Work out the finished part from the listing and answer in its coordinate system (mm). Face numbers are marked on the shaded views. A direction names the side the tool comes from. Give positions to 0.01 mm unless a question says otherwise; leave off trailing zeros. Order: outer loops, then holes, each group sorted by start corner. A loop starts at its lowest first (then second) coordinate and runs counter-clockwise, first axis right, second up. Notation, with made-up numbers: (38.25, -17) -> (79.25, -17) arc R29 ccw to (79.25, 12) -> close; hole circle Ø1 at (56.25, 59.5). An arc over 180 degrees is marked (long way). Answer as CSV lines item,"result". Start each with the question number.
1. For the marked faces 5 and 6, determine the directions among +Z, -Z, +X, -X, +Y, -Y from which every point of the face is accessible in a straight line to the end or side of a thin tool.
2. A cutting plane is placed at C-C (y = 35.5). Give the vertices of the cut face in (x, z) (3 decimals).
3. A cutting plane is placed at D-D (y = -38). Give the vertices of the cut face in (x, z) (3 decimals), then the cut area to 3 significant figures.
4. Find the intervals of material crossed by L1, parallel to X at y = -3, z = -2; L2, parallel to X at y = -0.5, z = -1.5; L3, parallel to Y at x = 4, z = -0.75, in increasing order.
5. For a pull along Y with two mould halves and no side action, classify the marked faces 1, 2, 3 and 4 as released by +Y, released by -Y, zero draft, split by the parting line, or undercut.
6. A cutting plane is placed at A-A (x = 0). Give the vertices of the cut face in (y, z) (3 decimals).
7. Flat-ended cylindrical pins translate along their axes: pin 1 (2 mm diameter, centred on x = -25, z = 1, fed in from +Y); pin 2 (3 mm diameter, centred on x = -1.5, z = 0, fed in from -Y); pin 3 (2 mm diameter, centred on x = 1.5, z = 1, fed in from +Y). Find the tip coordinate at first contact, or state that the pin passes through.
8. A cutting plane is placed at B-B (z = 2). Give the vertices of the cut face in (x, y), then the cut area to 3 significant figures.
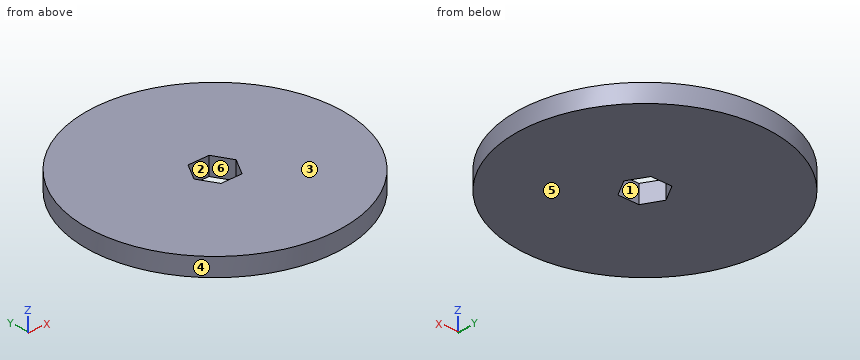
from build123d import *

# Parameters (mm, degrees)
SKETCH1_R           = 44.45
BOSS_EXTRUDE1_DEPTH = 3.175
CUT_EXTRUDE1_DEPTH  = 3.175


with BuildPart() as part:
    # Sketch1 → Boss-Extrude1 (new body, symmetric)
    with BuildSketch(Plane.XY):
        Circle(SKETCH1_R)
    extrude(amount=BOSS_EXTRUDE1_DEPTH, both=True)

    # Sketch2 → Cut-Extrude1 (cut, symmetric)
    with BuildSketch(Plane.XY):
        Polygon((7.332348419, 0), (3.666174209, 6.35), (-3.666174209, 6.35), (-7.332348419, 0), (-3.666174209, -6.35), (3.666174209, -6.35), align=None)
    extrude(amount=CUT_EXTRUDE1_DEPTH, both=True, mode=Mode.SUBTRACT)


solid = part.part
Answer sheet:
1,face 5,"-Z, +X, -X, +Y, -Y"
1,face 6,"+Z, -Z"
2,outline,"(-26.75, -3.175) -> (26.75, -3.175) -> (26.75, 3.175) -> (-26.75, 3.175) -> close"
3,outline,"(-23.061, -3.175) -> (23.061, -3.175) -> (23.061, 3.175) -> (-23.061, 3.175) -> close"
3,area,"293 mm^2"
4,L1,"x = -44.35 to -5.6, 5.6 to 44.35"
4,L2,"x = -44.45 to -7.04, 7.04 to 44.45"
4,L3,"y = -44.27 to -5.77, 5.77 to 44.27"
5,face 1,"undercut"
5,face 2,"undercut"
5,face 3,"zero draft"
5,face 4,"split by the parting line"
6,outline,"(-44.45, -3.175) -> (-6.35, -3.175) -> (-6.35, 3.175) -> (-44.45, 3.175) -> close; (6.35, -3.175) -> (44.45, -3.175) -> (44.45, 3.175) -> (6.35, 3.175) -> close"
7,pin 1,"stops at y = 37.41"
7,pin 2,"stops at y = -44.45"
7,pin 3,"stops at y = 44.45"
8,outline,"circle Ø88.9 at (0, 0); hole (-7.33, 0) -> (-3.67, -6.35) -> (3.67, -6.35) -> (7.33, 0) -> (3.67, 6.35) -> (-3.67, 6.35) -> close"
8,area,"6,070 mm^2"
